from build123d import *

# Parameters (mm, degrees)
SKETCH1_W           = 125.4
SKETCH1_H           = 125.4
BOSS_EXTRUDE1_DEPTH = 6.35
SKETCH4_W           = 6.35
SKETCH4_H           = 12.7
CUT_EXTRUDE1_DEPTH  = 7.35
SKETCH5_W           = 19.05
SKETCH5_H           = 6.35
CUT_EXTRUDE2_DEPTH  = 7.35
CIRPATTERN1_COUNT   = 4
CIRPATTERN2_COUNT   = 4


with BuildPart() as part:
    # Sketch1 → Boss-Extrude1 (new body)
    with BuildSketch(Plane(origin=(0, 0, 0), x_dir=(1, 0, 0), z_dir=(0, 1, 0))):
        Rectangle(SKETCH1_W, SKETCH1_H)
    extrude(amount=BOSS_EXTRUDE1_DEPTH)

    # Sketch4 → Cut-Extrude1 (cut, through all)
    with BuildSketch(Plane(origin=(0, 6.35, 0), x_dir=(1, 0, 0), z_dir=(0, 1, 0))):
        with Locations((-53.175, 43.65)):
            Rectangle(SKETCH4_W, SKETCH4_H)
    cut_extrude1 = extrude(amount=-CUT_EXTRUDE1_DEPTH, mode=Mode.SUBTRACT)

    # Sketch5 → Cut-Extrude2 (cut, through all)
    with BuildSketch(Plane(origin=(0, 6.35, 0), x_dir=(1, 0, 0), z_dir=(0, 1, 0))):
        with Locations((-46.825, 53.175)):
            Rectangle(SKETCH5_W, SKETCH5_H)
    cut_extrude2 = extrude(amount=-CUT_EXTRUDE2_DEPTH, mode=Mode.SUBTRACT)

    # CirPattern1: Cut-Extrude1 ×4 about axis
    cirpattern1_axis = Axis((0, 0, 0), (0, 1, 0))
    for i in range(1, CIRPATTERN1_COUNT):
        add(cut_extrude1.rotate(cirpattern1_axis, i * 360 / CIRPATTERN1_COUNT), mode=Mode.SUBTRACT)

    # CirPattern2: Cut-Extrude2 ×4 about axis
    cirpattern2_axis = Axis((0, 0, 0), (0, 1, 0))
    for i in range(1, CIRPATTERN2_COUNT):
        add(cut_extrude2.rotate(cirpattern2_axis, i * 360 / CIRPATTERN2_COUNT), mode=Mode.SUBTRACT)


solid = part.part
The listing builds one solid part. Answer for the finished solid, in the listing's coordinates (mm). A direction names the side the tool comes from. Coordinates: 2 decimals unless noted, no trailing zeros. Order: outer loops, then holes, each group sorted by start corner. A loop starts at its lowest first (then second) coordinate and runs counter-clockwise, first axis right, second up. Notation, with made-up numbers: M -12,32.25 L 10,32.25 A21 cw 10,54.25 Z; hole C 19,86.5 d8. An arc over 180 degrees is marked long. Use CSV: the item, a comma, the result in double quotes.
Q1. Straight lines are drawn through the part: L1, parallel to X at y = 3.5, z = -42; L2, parallel to Z at x = -53, y = 2.5. For each, find the intervals that lie inside material, in ascending order.
Here are the results:
L1,"-62.7 to -56.35, -50 to 50, 56.35 to 62.7"
L2,"-62.7 to -56.35, -37.3 to 37.3, 56.35 to 62.7"
Q2. A tool of negligible diameter and unlimited length cuts with its end or side. For faces 4 (the flat face through (53, 3, 37.3)), 5 (the flat face through (-1, 3, -62.7)), from which of +Z, -Z, +X, -X, +Y, -Y can it reach the whole face along a straight path? Write none if from no direction.
Here are the results:
face 4,"+Y, -Y"
face 5,"-Z, +X, -X, +Y, -Y"
Q3. Determine the mould class of faces 1 (the flat face through (-1, 0, -1)), 2 (the flat face through (-53, 3, 37.3)), 3 (the flat face through (-1, 3, 62.7)) for opening direction Z: pulls with the +Z half, pulls with the -Z half, needs draft (parallel to the pull), parting line crosses it, or undercut.
Here are the results:
face 1,"needs draft"
face 2,"undercut"
face 3,"pulls with the +Z half"
Q4. Section B-B (y = 1.5) is taken. Determine the outline of the cut face in (x, z).
Here are the results:
outline,"M -62.7,-62.7 L 62.7,-62.7 L 62.7,62.7 L -62.7,62.7 Z; hole M -56.35,-56.35 L -37.3,-56.35 L -37.3,-50 L -50,-50 L -50,-37.3 L -56.35,-37.3 Z; hole M -56.35,37.3 L -50,37.3 L -50,50 L -37.3,50 L -37.3,56.35 L -56.35,56.35 Z; hole M 37.3,-56.35 L 56.35,-56.35 L 56.35,-37.3 L 50,-37.3 L 50,-50 L 37.3,-50 Z; hole M 37.3,50 L 50,50 L 50,37.3 L 56.35,37.3 L 56.35,56.35 L 37.3,56.35 Z"
Q5. Section C-C (z = -53) is taken. Determine the outline of the cut face in (x, y).
Here are the results:
outline,"M -62.7,0 L -56.35,0 L -56.35,6.35 L -62.7,6.35 Z; M -37.3,0 L 37.3,0 L 37.3,6.35 L -37.3,6.35 Z; M 56.35,0 L 62.7,0 L 62.7,6.35 L 56.35,6.35 Z"
Q6. Section A-A (z = 43.5) is taken. Determine the outline of the cut face in (x, y), then the cut area to 3 significant figures.
Here are the results:
outline,"M -62.7,0 L -56.35,0 L -56.35,6.35 L -62.7,6.35 Z; M -50,0 L 50,0 L 50,6.35 L -50,6.35 Z; M 56.35,0 L 62.7,0 L 62.7,6.35 L 56.35,6.35 Z"
area,"716 mm2"
